```python
from build123d import *

# Parameters (mm, degrees)
F2_DEPTH = 12.5
F0_R     = 5
F3_DEPTH = 12.5


with BuildPart() as f2:
    # F1 (on Front) → F2 (new body, symmetric)
    with BuildSketch(Plane.XZ):
        with BuildLine():
            Line((-10, 0), (10, 0))
            Line((10, 0), (10, 12.0382448658))
            Line((10, 12.0382448658), (6.0506574175, 12.0382448658))
            ThreePointArc((6.0506574175, 12.0382448658), (0, 10), (-6.0506574175, 12.0382448658))
            Line((-6.0506574175, 12.0382448658), (-10, 12.0382448658))
            Line((-10, 12.0382448658), (-10, 0))
        make_face()
        with BuildLine():
            Line((10, 12.0382448658), (10, 0))
            Line((10, 0), (20, 0))
            add(Edge.make_bspline(
                [(14.5119228257, 12.0382448658), (16.3412818838, 8.2321157615), (18.1706409419, 4.1160578807), (20, 0)],
                knots=[0.8627980706, 0.8627980706, 0.8627980706, 0.8627980706, 1, 1, 1, 1], degree=3))
            Line((14.5119228257, 12.0382448658), (10, 12.0382448658))
        make_face()
        with BuildLine():
            Line((-20, 0), (-10, 0))
            Line((-10, 0), (-10, 12.0382448658))
            Line((-10, 12.0382448658), (-14.5119228257, 12.0382448658))
            add(Edge.make_bspline(
                [(-20, 0), (-18.1706409419, 4.1160578807), (-16.3412818838, 8.2321157615), (-14.5119228257, 12.0382448658)],
                knots=[0, 0, 0, 0, 0.1372019294, 0.1372019294, 0.1372019294, 0.1372019294], degree=3))
        make_face()
        with BuildLine():
            Line((6.0506574175, 12.0382448658), (10, 12.0382448658))
            Line((10, 12.0382448658), (10, 20))
            ThreePointArc((10, 20), (8.958419899, 15.556272633), (6.0506574175, 12.0382448658))
        make_face()
        with BuildLine():
            Line((10, 20), (10, 12.0382448658))
            Line((10, 12.0382448658), (14.5119228257, 12.0382448658))
            add(Edge.make_bspline(
                [(10, 20.625), (11.5039742752, 18.0870434106), (13.0079485504, 15.1673846789), (14.5119228257, 12.0382448658)],
                knots=[0.75, 0.75, 0.75, 0.75, 0.8627980706, 0.8627980706, 0.8627980706, 0.8627980706], degree=3))
            Line((10, 20.625), (10, 20))
        make_face()
        with BuildLine():
            Line((-14.5119228257, 12.0382448658), (-10, 12.0382448658))
            Line((-10, 12.0382448658), (-10, 20))
            Line((-10, 20), (-10, 20.625))
            add(Edge.make_bspline(
                [(-14.5119228257, 12.0382448658), (-13.0079485504, 15.1673846789), (-11.5039742752, 18.0870434106), (-10, 20.625)],
                knots=[0.1372019294, 0.1372019294, 0.1372019294, 0.1372019294, 0.25, 0.25, 0.25, 0.25], degree=3))
        make_face()
        with BuildLine():
            Line((-10, 20), (-10, 12.0382448658))
            Line((-10, 12.0382448658), (-6.0506574175, 12.0382448658))
            ThreePointArc((-6.0506574175, 12.0382448658), (-8.958419899, 15.556272633), (-10, 20))
        make_face()
        with BuildLine():
            ThreePointArc((6.0506574175, 12.0382448658), (8.958419899, 15.556272633), (10, 20))
            ThreePointArc((10, 20), (9.9945146107, 20.3311762316), (9.9780644607, 20.661989137))
            add(Edge.make_bspline(
                [(0, 30), (3.3260214869, 30), (6.6520429738, 26.2664336107), (9.9780644607, 20.661989137)],
                knots=[0.5, 0.5, 0.5, 0.5, 0.7494516115, 0.7494516115, 0.7494516115, 0.7494516115], degree=3))
            add(Edge.make_bspline(
                [(-9.9780644607, 20.661989137), (-6.6520429738, 26.2664336107), (-3.3260214869, 30), (0, 30)],
                knots=[0.2505483885, 0.2505483885, 0.2505483885, 0.2505483885, 0.5, 0.5, 0.5, 0.5], degree=3))
            ThreePointArc((-9.9780644607, 20.661989137), (-9.9945146107, 20.3311762316), (-10, 20))
            ThreePointArc((-10, 20), (-8.958419899, 15.556272633), (-6.0506574175, 12.0382448658))
            Line((-6.0506574175, 12.0382448658), (6.0506574175, 12.0382448658))
        make_face()
        with BuildLine():
            ThreePointArc((-6.0506574175, 12.0382448658), (0, 10), (6.0506574175, 12.0382448658))
            Line((6.0506574175, 12.0382448658), (-6.0506574175, 12.0382448658))
        make_face()
        with BuildLine():
            add(Edge.make_bspline(
                [(0, 30), (3.3260214869, 30), (6.6520429738, 26.2664336107), (9.9780644607, 20.661989137)],
                knots=[0.5, 0.5, 0.5, 0.5, 0.7494516115, 0.7494516115, 0.7494516115, 0.7494516115], degree=3))
            ThreePointArc((9.9780644607, 20.661989137), (6.8330120968, 27.301366015), (0, 30))
        make_face()
        with BuildLine():
            ThreePointArc((0, 30), (-6.8330120968, 27.301366015), (-9.9780644607, 20.661989137))
            add(Edge.make_bspline(
                [(-9.9780644607, 20.661989137), (-6.6520429738, 26.2664336107), (-3.3260214869, 30), (0, 30)],
                knots=[0.2505483885, 0.2505483885, 0.2505483885, 0.2505483885, 0.5, 0.5, 0.5, 0.5], degree=3))
        make_face()
    extrude(amount=F2_DEPTH, both=True)

    # F0 (on Front) → F3 (cut, symmetric)
    with BuildSketch(Plane.XZ):
        with Locations((0, 20)):
            Circle(F0_R)
    extrude(amount=F3_DEPTH, both=True, mode=Mode.SUBTRACT)


solid = f2.part
```
Verification items for the finished model (mm, model axes). Round coordinates to 2 decimals unless told otherwise and drop trailing zeros. Write each loop counter-clockwise with the first axis right and the second up, starting at its lowest first coordinate (ties: lowest second). Pieces come first, ordered by that corner, then holes. Notation, with made-up numbers: (52.5, 6.5) - (60.5, 6.5) arc R16 ccw to (60.5, 37.5) - close; hole circle Ø10 at (39.25, -23.5). An arc over 180 degrees is marked (long way). Answer as a JSON object with one key per item and string values. Group by question number.
Q1. Thickness scan on line 1 (X direction, y = -1.75, z = 16); line 2 (X direction, y = -9, z = 24.5); line 3 (Z direction, x = 1, y = -2). Record the ranges inside material, lowest first.
Q2. Go/stop test with flat-tipped pins: pin 1 Ø5 at (x, y) = (10, 9.5) entering from +Z; pin 2 Ø1.5 at (y, z) = (-1.5, 20.5) entering from -X; pin 3 Ø3 at (y, z) = (-4.5, 17) entering from +X. Record where each tip stops, or that it passes through.
Q3. Mould release check, pull along X, two halves, no side actions. Record for faces 1 (the cylindrical face through (-1.08, -0.18, 15.12)), 2 (the flat face through (0, 0, 0)): released by +X, released by -X, zero draft, split by the parting line, or undercut.
Q4. Section check C-C, the plane x = 9. Enter the section's corners in (y, z).
Q5. Section check A-A, the plane x = 0. Enter the section's corners in (y, z).
Q6. Section check B-B, the plane z = 22. Enter the section's corners in (x, y), plus the area to 3 significant figures.
Q7. Section check D-D, the plane z = 25.5. Enter the section's corners in (x, y).
Found:
{
 "1": {"line 1": "x = -12.54 to -3, 3 to 12.54", "line 2": "x = -8.93 to -2.18, 2.18 to 8.93", "line 3": "z = 0 to 15.1, 24.9 to 29.95"},
 "2": {"pin 1": "stops at z = 26.61", "pin 2": "stops at x = -10.51", "pin 3": "stops at x = 12.8"},
 "3": {"face 1": "undercut", "face 2": "zero draft"},
 "4": {"outline": "(-12.5, 0) - (12.5, 0) - (12.5, 24.36) - (-12.5, 24.36) - close"},
 "5": {"outline": "(-12.5, 0) - (12.5, 0) - (12.5, 15) - (-12.5, 15) - close; (-12.5, 25) - (12.5, 25) - (12.5, 30) - (-12.5, 30) - close"},
 "6": {"outline": "(-9.8, -12.5) - (-4.58, -12.5) - (-4.58, 12.5) - (-9.8, 12.5) - close; (4.58, -12.5) - (9.8, -12.5) - (9.8, 12.5) - (4.58, 12.5) - close", "area": "261 mm^2"},
 "7": {"outline": "(-8.35, -12.5) - (8.35, -12.5) - (8.35, 12.5) - (-8.35, 12.5) - close"}
}
